Work out the finished part from the listing and answer in its coordinate system (mm). A direction names the side the tool comes from. Round coordinates to 2 decimals unless told otherwise and drop trailing zeros. Write each loop counter-clockwise with the first axis right and the second up, starting at its lowest first coordinate (ties: lowest second). Pieces come first, ordered by that corner, then holes. Notation, with made-up numbers: (5, 16.5) -> (58, 16.5) arc R14 ccw to (58, 43.5) -> close; hole circle Ø9 at (-29, -5.5). An arc over 180 degrees is marked (long way). One line per item, written item: value.
```python
from build123d import *

# Parameters (mm, degrees)
F1_DEPTH = 3.175


with BuildPart() as f1:
    # F0 (on Top) → F1 (new body)
    with BuildSketch(Plane.XY):
        with BuildLine():
            ThreePointArc((5.908962, 8.264972), (3.102699, 9.67465), (0, 10.16))
            ThreePointArc((0, 10.16), (-3.102699, 9.67465), (-5.908962, 8.264972))
            Line((-5.908962, 8.264972), (-11.686093, 6.16389))
            Line((-11.686093, 6.16389), (-12.950189, 5.704151))
            ThreePointArc((-12.950189, 5.704151), (-15.547031, 3.361904), (-16.51, 0))
            ThreePointArc((-16.51, 0), (-15.547031, -3.361904), (-12.950189, -5.704151))
            Line((-12.950189, -5.704151), (-11.686093, -6.16389))
            Line((-11.686093, -6.16389), (-5.908962, -8.264972))
            ThreePointArc((-5.908962, -8.264972), (-3.102699, -9.67465), (0, -10.16))
            ThreePointArc((0, -10.16), (3.102699, -9.67465), (5.908962, -8.264972))
            Line((5.908962, -8.264972), (11.686093, -6.16389))
            Line((11.686093, -6.16389), (12.950189, -5.704151))
            ThreePointArc((12.950189, -5.704151), (15.547031, -3.361904), (16.51, 0))
            ThreePointArc((16.51, 0), (15.547031, 3.361904), (12.950189, 5.704151))
            Line((12.950189, 5.704151), (11.686093, 6.16389))
            Line((11.686093, 6.16389), (5.908962, 8.264972))
        make_face()
        with BuildLine():
            ThreePointArc((-6.35, 0), (-4.490128, 4.490128), (0, 6.35))
            ThreePointArc((0, 6.35), (1.502973, 6.169568), (2.920534, 5.638527))
            Line((2.920534, 5.638527), (2.920534, 0))
            Line((2.920534, 0), (2.920534, -5.638527))
            ThreePointArc((2.920534, -5.638527), (1.502973, -6.169568), (0, -6.35))
            ThreePointArc((0, -6.35), (-4.490128, -4.490128), (-6.35, 0))
        make_face(mode=Mode.SUBTRACT)
    extrude(amount=F1_DEPTH)


solid = f1.part
```
(1) Find section A-A on x = -5.5. Give the vertices of the cut face in (y, z) (3 decimals).
Reported:
outline: (-8.543, 0) -> (-3.174, 0) -> (-3.174, 3.175) -> (-8.543, 3.175) -> close; (3.174, 0) -> (8.543, 0) -> (8.543, 3.175) -> (3.174, 3.175) -> close
(2) Consider probe 1 along X at (y, z) = (0.75, 0.25); probe 2 along Y at (x, z) = (-3.5, 0.8); probe 3 along Y at (x, z) = (-3, 1.35). Determine where each line is inside the solid, lowest interval first.
Reported:
probe 1: x = -16.47 to -6.31, 2.92 to 16.47
probe 2: y = -9.54 to -5.3, 5.3 to 9.54
probe 3: y = -9.71 to -5.6, 5.6 to 9.71
(3) A tool of negligible diameter and unlimited length cuts with its end or side. For faces 4 (the face through (3.4, 0.1, 0)), 5 (the face through (1.524, -6.165, 1.565)), from which of +Z, -Z, +X, -X, +Y, -Y can it reach the whole face along a straight path? Write none if from no direction.
Reported:
face 4: -Z, +X, -X, +Y, -Y
face 5: +Z, -Z
(4) Find section C-C on y = 4.25. Give the vertices of the cut face in (x, z) (3 decimals).
Reported:
outline: (-14.878, 0) -> (-4.718, 0) -> (-4.718, 3.175) -> (-14.878, 3.175) -> close; (2.921, 0) -> (14.878, 0) -> (14.878, 3.175) -> (2.921, 3.175) -> close
(5) Find section D-D on y = -7. Give the vertices of the cut face in (x, z) (3 decimals).
Reported:
outline: (-9.387, 0) -> (9.387, 0) -> (9.387, 3.175) -> (-9.387, 3.175) -> close
(6) Flat-ended cylindrical pins translate along their axes: pin 1 Ø3 at (x, y) = (6, -0.5) entering from -Z; pin 2 Ø1.6 at (y, z) = (-2.5, 2.5) entering from -X. Find the tip coordinate at first contact, or state that the pin passes through.
Reported:
pin 1: stops at z = 0
pin 2: stops at x = -16.28
(7) Find section B-B on z = 0.9. Give the vertices of the cut face in (x, y), plus the area to 3 significant figures.
Reported:
outline: (-16.51, 0) arc R6.35 ccw to (-12.95, -5.7) -> (-11.69, -6.16) -> (-5.91, -8.26) arc R10.16 ccw to (0, -10.16) arc R10.16 ccw to (5.91, -8.26) -> (11.69, -6.16) -> (12.95, -5.7) arc R6.35 ccw to (16.51, 0) arc R6.35 ccw to (12.95, 5.7) -> (11.69, 6.16) -> (5.91, 8.26) arc R10.16 ccw to (0, 10.16) arc R10.16 ccw to (-5.91, 8.26) -> (-11.69, 6.16) -> (-12.95, 5.7) arc R6.35 ccw to start; hole (0, -6.35) arc R6.35 ccw to (2.92, -5.64) -> (2.92, 5.64) arc R6.35 ccw to (0, 6.35) arc R6.35 ccw to start
area: 382 mm2
(8) For a pull along X with two mould halves and no side action, classify faces 1 (the face through (1.482, 6.175, 1.565)), 2 (the face through (3.4, 0.1, 3.175)), 3 (the face through (2.921, 0, 2)) as pulls with the +X half, pulls with the -X half, needs draft (parallel to the pull), parting line crosses it, or undercut.
Reported:
face 1: undercut
face 2: needs draft
face 3: undercut
